Geometry: final body of the model. Coordinates: model frame, mm. Round coordinates to 2 decimals unless told otherwise and drop trailing zeros. Loops run counter-clockwise (first coordinate to the right, second up) from the corner with the lowest first, then second, coordinate; pieces in that order, holes last. Notation, with made-up numbers: (79, 61.25) -> (84, 61.25) arc R30 cw to (84, 96.25) -> close; hole circle Ø5 at (62.5, 66). An arc over 180 degrees is marked (long way). Answer in a Markdown table with one row per item.
```python
from build123d import *

# Parameters (mm, degrees)
SKETCH1_W           = 350
SKETCH1_H           = 230
BOSS_EXTRUDE1_DEPTH = 20
CUT_EXTRUDE1_DEPTH  = 5
SKETCH4_R           = 15
CUT_EXTRUDE2_DEPTH  = 20


with BuildPart() as part:
    # Sketch1 → Boss-Extrude1 (new body)
    with BuildSketch(Plane.XY):
        with Locations((11.12716763, -28.294797688)):
            Rectangle(SKETCH1_W, SKETCH1_H)
    extrude(amount=BOSS_EXTRUDE1_DEPTH)

    # Sketch3 → Cut-Extrude1 (cut)
    with BuildSketch(Plane.XY.offset(20)):
        with BuildLine():
            Line((-125.87283237, -24.794797688), (-93.87283237, -24.794797688))
            Line((-93.87283237, -24.794797688), (-93.87283237, 5.205202312))
            Line((-93.87283237, 5.205202312), (-83.87283237, 5.205202312))
            Line((-83.87283237, 5.205202312), (-83.87283237, -24.794797688))
            Line((-83.87283237, -24.794797688), (6.12716763, -24.794797688))
            Line((6.12716763, -24.794797688), (6.12716763, 5.205202312))
            Line((6.12716763, 5.205202312), (16.12716763, 5.205202312))
            Line((16.12716763, 5.205202312), (16.12716763, -24.794797688))
            Line((16.12716763, -24.794797688), (106.12716763, -24.794797688))
            Line((106.12716763, -24.794797688), (106.12716763, 5.205202312))
            Line((106.12716763, 5.205202312), (116.12716763, 5.205202312))
            Line((116.12716763, 5.205202312), (116.12716763, -24.794797688))
            Line((116.12716763, -24.794797688), (148.12716763, -24.794797688))
            ThreePointArc((148.12716763, -24.794797688), (150.248487974, -25.673477344), (151.12716763, -27.794797688))
            Line((151.12716763, -27.794797688), (151.12716763, -28.794797688))
            ThreePointArc((151.12716763, -28.794797688), (150.248487974, -30.916118031), (148.12716763, -31.794797688))
            Line((148.12716763, -31.794797688), (116.12716763, -31.794797688))
            Line((116.12716763, -31.794797688), (116.12716763, -61.794797688))
            Line((116.12716763, -61.794797688), (106.12716763, -61.794797688))
            Line((106.12716763, -61.794797688), (106.12716763, -31.794797688))
            Line((106.12716763, -31.794797688), (16.12716763, -31.794797688))
            Line((16.12716763, -31.794797688), (16.12716763, -61.794797688))
            Line((16.12716763, -61.794797688), (6.12716763, -61.794797688))
            Line((6.12716763, -61.794797688), (6.12716763, -31.794797688))
            Line((6.12716763, -31.794797688), (-83.87283237, -31.794797688))
            Line((-83.87283237, -31.794797688), (-83.87283237, -61.794797688))
            Line((-83.87283237, -61.794797688), (-93.87283237, -61.794797688))
            Line((-93.87283237, -61.794797688), (-93.87283237, -31.794797688))
            Line((-93.87283237, -31.794797688), (-125.87283237, -31.794797688))
            ThreePointArc((-125.87283237, -31.794797688), (-127.994152714, -30.916118031), (-128.87283237, -28.794797688))
            Line((-128.87283237, -28.794797688), (-128.87283237, -27.794797688))
            ThreePointArc((-128.87283237, -27.794797688), (-127.994152714, -25.673477344), (-125.87283237, -24.794797688))
        make_face()
    extrude(amount=-CUT_EXTRUDE1_DEPTH, mode=Mode.SUBTRACT)

    # Sketch4 → Cut-Extrude2 (cut)
    with BuildSketch(Plane.XY.offset(20)):
        with Locations((111.12716763, 15.205202312)):
            Circle(SKETCH4_R)
        with Locations((11.12716763, 15.205202312)):
            Circle(SKETCH4_R)
        with Locations((-88.87283237, 15.205202312)):
            Circle(SKETCH4_R)
        with Locations((111.12716763, -71.794797688)):
            Circle(SKETCH4_R)
        with Locations((11.12716763, -71.794797688)):
            Circle(SKETCH4_R)
        with Locations((-88.87283237, -71.794797688)):
            Circle(SKETCH4_R)
    extrude(amount=-CUT_EXTRUDE2_DEPTH, mode=Mode.SUBTRACT)


solid = part.part
```
Item 1: Cut plane B-B (z = 6.5). Output: boundary loops of the cut face in (x, y).
Answer:
| item | result |
|---|---|
| outline | (-163.87, -143.29) -> (186.13, -143.29) -> (186.13, 86.71) -> (-163.87, 86.71) -> close; hole circle Ø30 at (-88.87, -71.79); hole circle Ø30 at (-88.87, 15.21); hole circle Ø30 at (11.13, -71.79); hole circle Ø30 at (11.13, 15.21); hole circle Ø30 at (111.13, -71.79); hole circle Ø30 at (111.13, 15.21) |
Item 2: Draft query along X for faces 1 (the face through (19.191, 27.853, 10.14)), 2 (the face through (-163.873, -30, 10)), 3 (the face through (186.127, -30, 10)), 4 (the face through (9, -27, 0)). Return one class per face: pulls with the +X half, pulls with the -X half, needs draft (parallel to the pull), parting line crosses it, or undercut.
Answer:
| item | result |
|---|---|
| face 1 | undercut |
| face 2 | pulls with the -X half |
| face 3 | pulls with the +X half |
| face 4 | needs draft |
Item 3: Cut plane C-C (y = -79.5). Output: boundary loops of the cut face in (x, z), then the cut area to 3 significant figures.
Answer:
| item | result |
|---|---|
| outline | (-163.87, 0) -> (-101.74, 0) -> (-101.74, 20) -> (-163.87, 20) -> close; (-76, 0) -> (-1.74, 0) -> (-1.74, 20) -> (-76, 20) -> close; (24, 0) -> (98.26, 0) -> (98.26, 20) -> (24, 20) -> close; (124, 0) -> (186.13, 0) -> (186.13, 20) -> (124, 20) -> close |
| area | 5,460 mm² |
Item 4: Cut plane A-A (y = -8). Output: boundary loops of the cut face in (x, z), then the cut area to 3 significant figures.
Answer:
| item | result |
|---|---|
| outline | (-163.87, 0) -> (186.13, 0) -> (186.13, 20) -> (116.13, 20) -> (116.13, 15) -> (106.13, 15) -> (106.13, 20) -> (16.13, 20) -> (16.13, 15) -> (6.13, 15) -> (6.13, 20) -> (-83.87, 20) -> (-83.87, 15) -> (-93.87, 15) -> (-93.87, 20) -> (-163.87, 20) -> close |
| area | 6,850 mm² |
Item 5: Line query: probe 1 along Y at (x, z) = (-38.5, 18); probe 2 along X at (y, z) = (-85.5, 15.75); probe 3 along X at (y, z) = (13, 5.25). Output: solid intervals per line, ascending. Write a range as [from, to].
Answer:
| item | result |
|---|---|
| probe 1 | y = [-143.29, -31.79], [-24.79, 86.71] |
| probe 2 | x = [-163.87, -94.97], [-82.78, 5.03], [17.22, 105.03], [117.22, 186.13] |
| probe 3 | x = [-163.87, -103.71], [-74.04, -3.71], [25.96, 96.29], [125.96, 186.13] |
Item 6: Pin query (flat end, axial travel): pin 1 Ø18 at (x, y) = (111.13, 15.21) entering from -Z. Return the tip coordinate at first contact, or that it passes through.
Answer:
| item | result |
|---|---|
| pin 1 | passes through |
